Autodesk Inventor part; units mm, degrees
ref_plane "YZ Plane" through (0, 0, 0) normal (1, 0, 0) x (0, 1, 0)
ref_plane "XZ Plane" through (0, 0, 0) normal (0, 1, 0) x (-1, 0, 0)
ref_plane "XY Plane" through (0, 0, 0) normal (0, 0, 1) x (1, 0, 0)
sketch "Sketch1" plane through (0, 0, 0) normal (0, 0, 1) x (1, 0, 0)
  line L0 (-30, 29) -> (30, 29)
  line L1 (40, 19) -> (40, -19)
  line L2 (30, -29) -> (-30, -29)
  line L3 (-40, -19) -> (-40, 19)
  arc A0 (-30, 29) -> (-40, 19) centre (-30, 19) ccw
  arc A1 (40, 19) -> (30, 29) centre (30, 19) ccw
  arc A2 (-40, -19) -> (-30, -29) centre (-30, -19) ccw
  arc A3 (30, -29) -> (40, -19) centre (30, -19) ccw
  line L4 (-10, 24) -> (10, 24)
  line L5 (10, 24) -> (10, 16.5)
  line L6 (10, 16.5) -> (-10, 16.5)
  line L7 (-10, 16.5) -> (-10, 24)
  point P0 (0, 0)
  point P1 (-40, 29)
  point P2 (40, -29)
  point P3 (40, 29)
  point P4 (-40, -29)
  point P5 (40, 0)
  point P6 (0, 29)
  point P7 (0, 16.5)
  dimension "d0" = 58
  dimension "d1" = 80
  dimension "d4" = 10
  dimension "d13" = 5
  dimension "d14" = 7.5
  dimension "d15" = 20
extrude "Extrusion1" add sketch "Sketch1" along normal blind 3
sketch "Sketch2" plane through (0, 0, 3) normal (0, 0, 1) x (1, 0, 0)
  line L0 (30, 29) -> (-30, 29)
  arc A0 (-30, 29) -> (-40, 19) centre (-30, 19) ccw
  line L1 (-40, 19) -> (-40, -19)
  arc A1 (-40, -19) -> (-30, -29) centre (-30, -19) ccw
  line L2 (-30, -29) -> (30, -29)
  arc A2 (30, -29) -> (40, -19) centre (30, -19) ccw
  line L3 (40, -19) -> (40, 19)
  arc A3 (40, 19) -> (30, 29) centre (30, 19) ccw
  line L4 (-32.5, -18) -> (-29.5, -18)
  line L5 (-29.5, -18) -> (-29.5, -12)
  line L6 (-29.5, -12) -> (-32.5, -12)
  line L7 (-32.5, -12) -> (-32.5, -18)
  line L8 (-32.5, 6) -> (-29.5, 6)
  line L9 (-29.5, 6) -> (-29.5, 12)
  line L10 (-29.5, 12) -> (-32.5, 12)
  line L11 (-32.5, 12) -> (-32.5, 6)
  line L12 (29.5, -18) -> (32.5, -18)
  line L13 (32.5, -18) -> (32.5, -12)
  line L14 (32.5, -12) -> (29.5, -12)
  line L15 (29.5, -12) -> (29.5, -18)
  line L16 (29.5, 6) -> (32.5, 6)
  line L17 (32.5, 6) -> (32.5, 12)
  line L18 (32.5, 12) -> (29.5, 12)
  line L19 (29.5, 12) -> (29.5, 6)
  line L20 (-31, 6) -> (-31, -12) construction
  point P0 (0, 0)
  point P1 (-31, -3)
  point P2 (31, -3)
  point P3 (31, 6)
  point P4 (-31, -3)
  dimension "d5" = 62
  dimension "d17" = 31
  dimension "d18" = 3
  dimension "d19" = 6
  dimension "d20" = 3
  dimension "d21" = 18
hole "Hole1" at (-31, -3, 3) at (31, -3, 3) direction (0, 0, -1) diameter 3 end through all
extrude "Extrusion2" cut sketch "Sketch2" against normal up to next contours L7 L6 L5 L4 | L11 L10 L9 L8 | L15 L14 L13 L12 | L19 L18 L17 L16
properties part number "Front_panel" material "Polycarbonate, Clear"
Input: part model. Units: mm. Frame: model coordinates. A direction names the side the tool comes from. Round coordinates to 2 decimals unless told otherwise and drop trailing zeros. Write each loop counter-clockwise with the first axis right and the second up, starting at its lowest first coordinate (ties: lowest second). Pieces come first, ordered by that corner, then holes.
1) Contact query for a flat-ended pin moving along its axis: P1, Ø1.5, axis at x = 31, z = 2, coming from the -Y side. Output: stop coordinate, or through.
2) Cut plane C-C (x = -31). Return the cut outline in (y, z), then the cut area to 3 significant figures.
3) Reachability of faces 1 (the flat face through (-29.5, 9, 2)), 2 (the flat face through (0, 29, 1)) from +Z, -Z, +X, -X, +Y, -Y: full face, straight path, thin tool, end or side. Return the list, or none.
4) Ray query, L1, parallel to X at y = -3, z = 2; L2, parallel to Y at x = -4, z = 1.9; L3, parallel to Y at x = 31, z = 1.6. Return the intervals inside material, ascending.
5) Cut plane B-B (z = 0.6). Count the separate pieces of the cut face and the enclosed holes in it, then the cut area to 3 significant figures.
6) Draft query along Y for faces 3 (the flat face through (-1, 0, 0)), 4 (the flat face through (-31, -18, 2)), 5 (the cylindrical face through (37.15, -25.99, 1.48)). Return one class per face: pulls with the +Y half, pulls with the -Y half, needs draft (parallel to the pull), parting line crosses it, or undercut.
7) Cut plane A-A (y = 11). Return the cut outline in (x, z).
Geometry says:
1. P1: stops at y = -29
2. outline: (-28.95, 0) - (-18, 0) - (-18, 3) - (-28.95, 3) - close; (-12, 0) - (-4.5, 0) - (-4.5, 3) - (-12, 3) - close; (-1.5, 0) - (6, 0) - (6, 3) - (-1.5, 3) - close; (12, 0) - (28.95, 0) - (28.95, 3) - (12, 3) - close
2. area: 129 mm2
3. face 1: +Z, -Z
3. face 2: +Z, -Z, +X, -X, +Y
4. L1: x = -40 to -32.5, -29.5 to 29.5, 32.5 to 40
4. L2: y = -29 to 16.5, 24 to 29
4. L3: y = -28.95 to -18, -12 to -4.5, -1.5 to 6, 12 to 28.95
5. separate pieces: 1
5. enclosed holes: 7
5. area: 4,320 mm2
6. face 3: needs draft
6. face 4: undercut
6. face 5: pulls with the -Y half
7. outline: (-40, 0) - (-32.5, 0) - (-32.5, 3) - (-40, 3) - close; (-29.5, 0) - (29.5, 0) - (29.5, 3) - (-29.5, 3) - close; (32.5, 0) - (40, 0) - (40, 3) - (32.5, 3) - close
